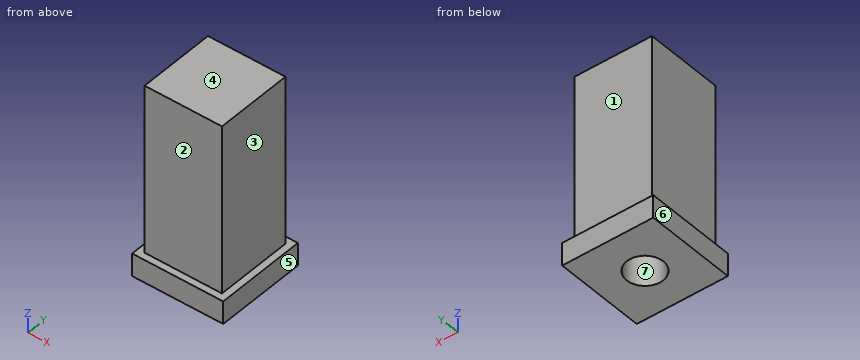
from build123d import *

# Parameters (mm, degrees)
SKETCH_1_W          = 20
SKETCH_1_H          = 20
EXTRUDE_1_DEPTH     = 5
SKETCH_2_W          = 17
SKETCH_2_H          = 17
EXTRUDE_2_DEPTH     = 37
SKETCH_3_R          = 4
CUT_EXTRUDE_1_DEPTH = 10


with BuildPart() as part:
    # ｽｹｯﾁ1 → ﾎﾞｽ - 押し出し1 (new body)
    with BuildSketch(Plane.XY):
        Rectangle(SKETCH_1_W, SKETCH_1_H)
    extrude(amount=EXTRUDE_1_DEPTH)

    # ｽｹｯﾁ2 → ﾎﾞｽ - 押し出し2 (add)
    with BuildSketch(Plane.XY.offset(5)):
        Rectangle(SKETCH_2_W, SKETCH_2_H)
    extrude(amount=EXTRUDE_2_DEPTH)

    # ｽｹｯﾁ3 → ｶｯﾄ - 押し出し1 (cut)
    with BuildSketch(Plane(origin=(0, 0, 0), x_dir=(-1, 0, 0), z_dir=(0, 0, -1))):
        Circle(SKETCH_3_R)
    extrude(amount=-CUT_EXTRUDE_1_DEPTH, mode=Mode.SUBTRACT)


solid = part.part
Verification items for the finished model (mm, model axes). Face numbers are marked on the shaded views. A direction names the side the tool comes from. Coordinates: 2 decimals unless noted, no trailing zeros. Write each loop counter-clockwise with the first axis right and the second up, starting at its lowest first coordinate (ties: lowest second). Pieces come first, ordered by that corner, then holes. Notation, with made-up numbers: (-27, -25) - (24, -25) arc R25 ccw to (24, 8) - close; hole circle Ø3 at (48, 50). An arc over 180 degrees is marked (long way). Answer as a JSON object with one key per item and string values.
(1) Cross-section at A-A on x = -5.25. Record the cut outline in (y, z).
Report:
{"outline": "(-10, 0) - (10, 0) - (10, 5) - (8.5, 5) - (8.5, 42) - (-8.5, 42) - (-8.5, 5) - (-10, 5) - close"}
(2) Tool access check on the marked faces 1, 2 and 3. Record the directions out of +Z, -Z, +X, -X, +Y, -Y that give a thin tool (end or side, any length) a straight path to the whole face; none if there is none.
Report:
{"face 1": "+Z, +X, -X, +Y", "face 2": "+Z, +X, -X, -Y", "face 3": "+Z, +X, +Y, -Y"}
(3) Cross-section at C-C on z = 11.5. Record the cut outline in (x, y).
Report:
{"outline": "(-8.5, -8.5) - (8.5, -8.5) - (8.5, 8.5) - (-8.5, 8.5) - close"}
(4) Mould release check, pull along X, two halves, no side actions. Record for the marked faces 4, 5, 6 and 7: pulls with the +X half, pulls with the -X half, needs draft (parallel to the pull), parting line crosses it, or undercut.
Report:
{"face 4": "needs draft", "face 5": "pulls with the +X half", "face 6": "pulls with the -X half", "face 7": "undercut"}
(5) Cross-section at B-B on y = 0. Record the cut outline in (x, z).
Report:
{"outline": "(-10, 0) - (-4, 0) - (-4, 10) - (4, 10) - (4, 0) - (10, 0) - (10, 5) - (8.5, 5) - (8.5, 42) - (-8.5, 42) - (-8.5, 5) - (-10, 5) - close"}
(6) Thickness scan on line 1 along Y through (x, z) = (0, 8.25); line 2 along X through (y, z) = (-0.75, 13). Record the ranges inside material, lowest first.
Report:
{"line 1": "-8.5 to -4, 4 to 8.5", "line 2": "-8.5 to 8.5"}
(7) Gauge pin test, flat ends, axial feed: pin 1 Ø2 at (y, z) = (4.5, 31) entering from -X; pin 2 Ø4 at (x, y) = (-1, 0) entering from -Z; pin 3 Ø8.5 at (y, z) = (-2.5, 18) entering from +X; pin 4 Ø5 at (x, y) = (1.5, 2) entering from -Z. Record the tip position at first contact, or that the pin passes through.
Report:
{"pin 1": "x = -8.5", "pin 2": "z = 10", "pin 3": "x = 8.5", "pin 4": "z = 0"}
